```python
from build123d import *

# Parameters (mm, degrees)
SKETCH1_R          = 20.5
SKETCH1_R_2        = 10
SKETCH1_R_3        = 1.651
EXTRUDE1_DEPTH     = 0.254
CUT_EXTRUDE1_DEPTH = 29.992490683
CIRPATTERN1_COUNT  = 3


with BuildPart() as part:
    # Sketch1 → Extrude1 (new body)
    with BuildSketch(Plane.XY):
        Circle(SKETCH1_R)
        Circle(SKETCH1_R_2, mode=Mode.SUBTRACT)
        with Locations((0, 16.5)):
            Circle(SKETCH1_R_3, mode=Mode.SUBTRACT)
        with Locations((14.289419162, -8.25)):
            Circle(SKETCH1_R_3, mode=Mode.SUBTRACT)
        with Locations((-14.289419162, -8.25)):
            Circle(SKETCH1_R_3, mode=Mode.SUBTRACT)
    extrude(amount=EXTRUDE1_DEPTH)

    # Sketch4 → Cut-Extrude1 (cut, through all)
    with BuildSketch(Plane(origin=(0, 0, 0), x_dir=(-1, 0, 0), z_dir=(0, 0, -1))):
        with BuildLine():
            ThreePointArc((1.5, -16.5), (0, -15), (-1.5, -16.5))
            Line((-1.5, -16.5), (-1.5, -20.4450483))
            ThreePointArc((-1.5, -20.4450483), (0, -20.5), (1.5, -20.4450483))
            Line((1.5, -20.4450483), (1.5, -16.5))
        make_face()
    cut_extrude1 = extrude(amount=-CUT_EXTRUDE1_DEPTH, mode=Mode.SUBTRACT)

    # CirPattern1: Cut-Extrude1 ×3 about axis
    cirpattern1_axis = Axis((0, 0, 0), (0, 0, 1))
    for i in range(1, CIRPATTERN1_COUNT):
        add(cut_extrude1.rotate(cirpattern1_axis, i * 360 / CIRPATTERN1_COUNT), mode=Mode.SUBTRACT)


solid = part.part
```
Input: part model. Units: mm. Frame: model coordinates. Give positions to 0.01 mm unless a question says otherwise; leave off trailing zeros. Order: outer loops, then holes, each group sorted by start corner. A loop starts at its lowest first (then second) coordinate and runs counter-clockwise, first axis right, second up. Notation, with made-up numbers: M -26.75,65.25 L -13.75,65.25 A26 ccw -13.75,89.25 Z; hole C 38.5,-27 d9. An arc over 180 degrees is marked long. Return JSON: item names as keys, results as strings.
Item 1: Ray query, probe 1 along Y at (x, z) = (0, 0.2); probe 2 along X at (y, z) = (-2, 0.15); probe 3 along Y at (x, z) = (11.5, 0.15). Return the intervals inside material, ascending.
Solutions:
{"probe 1": "-15 to -10, 10 to 14.85, 18.15 to 20.5", "probe 2": "-20.4 to -9.8, 9.8 to 20.4", "probe 3": "-16.97 to 16.97"}
Item 2: Cut plane D-D (y = -8.25). Return loops of the section in (x, z), then the cut area to 3 significant figures.
Solutions:
{"outline": "M -18.77,0 L -15.94,0 L -15.94,0.25 L -18.77,0.25 Z; M -12.64,0 L -5.65,0 L -5.65,0.25 L -12.64,0.25 Z; M 5.65,0 L 12.64,0 L 12.64,0.25 L 5.65,0.25 Z; M 15.94,0 L 18.77,0 L 18.77,0.25 L 15.94,0.25 Z", "area": "4.99 mm^2"}
Item 3: Cut plane A-A (y = 0). Return loops of the section in (x, z).
Solutions:
{"outline": "M -20.5,0 L -10,0 L -10,0.25 L -20.5,0.25 Z; M 10,0 L 20.5,0 L 20.5,0.25 L 10,0.25 Z"}
Item 4: Cut plane C-C (x = 2.5). Return loops of the section in (y, z).
Solutions:
{"outline": "M -20.35,0 L -9.68,0 L -9.68,0.25 L -20.35,0.25 Z; M 9.68,0 L 20.35,0 L 20.35,0.25 L 9.68,0.25 Z"}
Item 5: Cut plane B-B (z = 0.05). Return loops of the section in (x, y), then the cut area to 3 significant figures.
Solutions:
{"outline": "M -18.46,8.92 A20.5 ccw -1.5,-20.45 L -1.5,-16.5 A1.5 cw 1.5,-16.5 L 1.5,-20.45 A20.5 ccw 18.46,8.92 L 15.04,6.95 A1.5 cw 13.54,9.55 L 16.96,11.52 A20.5 ccw -16.96,11.52 L -13.54,9.55 A1.5 cw -15.04,6.95 Z; hole C -14.29,-8.25 d3.3; hole C 0,0 d20; hole C 0,16.5 d3.3; hole C 14.29,-8.25 d3.3", "area": "934 mm^2"}
Item 6: First-contact query: P1, Ø4, axis at x = 14.29, y = -8.25, coming from the -Z side. Flat tip, straight axial feed; report the tip coordinate or a pass-through.
Solutions:
{"P1": "z = 0"}
